```python
from build123d import *

# Parameters (mm, degrees)
F0_W      = 20
F0_H      = 5
F1_DEPTH  = 2
F2_R      = 2
F3_W      = 16
F3_H      = 2
F4_DEPTH  = 4
F5_R      = 2
F6_R      = 0.5
F7_DEPTH  = 2.001
F8_R      = 1.376408
F9_DEPTH  = 2.001
F11_W     = 1.233603
F11_H     = 9
F10_W     = 1.27
F10_H     = 9
F12_DEPTH = 0.635


with BuildPart() as f1:
    # F0 (on Top) → F1 (new body)
    with BuildSketch(Plane.XY):
        Rectangle(F0_W, F0_H)
    extrude(amount=F1_DEPTH)

    # F2
    f2_edges = [f1.edges().sort_by_distance(p)[0] for p in [
        (-10, -2.5, 1),
        (-10, 2.5, 1),
        (10, 2.5, 1),
        (10, -2.5, 1),
    ]]
    fillet(f2_edges, radius=F2_R)

    # F3 (on face) → F4 (join)
    with BuildSketch(Plane(origin=(0, 2.5, 0), x_dir=(-1, 0, 0), z_dir=(0, 1, 0))):
        with Locations((0, 1)):
            Rectangle(F3_W, F3_H)
    extrude(amount=F4_DEPTH)

    # F5
    f5_edges = [f1.edges().sort_by_distance(p)[0] for p in [
        (-8, 6.5, 1),
        (8, 6.5, 1),
    ]]
    fillet(f5_edges, radius=F5_R)

    # F6 (on face) → F7 (cut, through all)
    with BuildSketch(Plane.XY.offset(2)):
        Circle(F6_R)
        with Locations((-5, 0)):
            Circle(F6_R)
        with Locations((5, 0)):
            Circle(F6_R)
    extrude(amount=-F7_DEPTH, mode=Mode.SUBTRACT)

    # F8 (on face) → F9 (cut, through all)
    with BuildSketch(Plane.XY.offset(2)):
        with Locations((-7.627351, 0)):
            Circle(F8_R)
        with Locations((7.627366, 0)):
            Circle(F8_R)
        with Locations((-5, 3.96)):
            Circle(F8_R)
        with Locations((0, 3.96)):
            Circle(F8_R)
        with Locations((5, 3.96)):
            Circle(F8_R)
    extrude(amount=-F9_DEPTH, mode=Mode.SUBTRACT)

    # F11 (on face) + F10 (on face) → F12 (cut)
    with BuildSketch(Plane.XY.offset(2)):
        with Locations((-2.538401, 2)):
            Rectangle(F11_W, F11_H)
    with BuildSketch(Plane.XY.offset(2)):
        with Locations((2.54, 2)):
            Rectangle(F10_W, F10_H)
    extrude(amount=-F12_DEPTH, mode=Mode.SUBTRACT)


solid = f1.part
```
Geometry check sheet. Reference: the model listing, model coordinates, mm. A direction names the side the tool comes from. Give positions to 0.01 mm unless a question says otherwise; leave off trailing zeros. Loops run counter-clockwise (first coordinate to the right, second up) from the corner with the lowest first, then second, coordinate; pieces in that order, holes last. Notation, with made-up numbers: M -37,-4 L 14,-4 A31 cw 14,28 Z; hole C 25.25,74 d8. An arc over 180 degrees is marked long. Answer as CSV lines item,"result".
Item 1: Depth check by flat-ended pin: P1, Ø2, axis at x = 0, y = 3.96, coming from the -Z side; P2, Ø0.6, axis at y = 4, z = 1, coming from the +X side; P3, Ø1, axis at y = 4, z = 0.5, coming from the -X side. Enter the tip coordinate at first touch or a pass-through.
Values:
P1,"passes through"
P2,"stops at x = 8"
P3,"stops at x = -8"
Item 2: Access from +Z, -Z, +X, -X, +Y, -Y to the whole of each face (thin tool, end or side, straight path). Record for faces 1 (the cylindrical face through (8.899, -0.527, 1.014)), 2 (the flat face through (3, 2, 1.365)).
Values:
face 1,"+Z, -Z"
face 2,"+Z, +Y, -Y"
Item 3: Release check for a two-part mould opening along X. For faces 3 (the cylindrical face through (-0.298, 2.616, 1.014)), 4 (the cylindrical face through (-0.108, -0.488, 1.014)), 5 (the flat face through (-10, 0, 1)), 6 (the flat face through (0, -2.5, 1)) record: pulls with the +X half, pulls with the -X half, needs draft (parallel to the pull), parting line crosses it, or undercut.
Values:
face 3,"undercut"
face 4,"undercut"
face 5,"pulls with the -X half"
face 6,"needs draft"
Item 4: Cross-section at B-B on x = -5. Record the cut outline in (y, z).
Values:
outline,"M -2.5,0 L -0.5,0 L -0.5,2 L -2.5,2 Z; M 0.5,0 L 2.58,0 L 2.58,2 L 0.5,2 Z; M 5.34,0 L 6.5,0 L 6.5,2 L 5.34,2 Z"
Item 5: Cross-section at C-C on y = 0. Count the separate pieces of the cut face and the enclosed holes in it, and give its area (3 significant figures).
Values:
separate pieces,"6"
enclosed holes,"0"
area,"21.4 mm²"
Item 6: Material ranges on line 1 (Y direction, x = -5, z = 1.2); line 2 (Y direction, x = -5.25, z = 0.3); line 3 (X direction, y = 3.75, z = 0.45), recorded low to high.
Values:
line 1,"y = -2.5 to -0.5, 0.5 to 2.58, 5.34 to 6.5"
line 2,"y = -2.5 to -0.43, 0.43 to 2.61, 5.31 to 6.5"
line 3,"x = -8 to -6.36, -3.64 to -1.36, 1.36 to 3.64, 6.36 to 8"
Item 7: Cross-section at A-A on y = 3.96. Record the cut outline in (x, z) (3 decimals).
Values:
outline,"M -8,0 L -6.376,0 L -6.376,2 L -8,2 Z; M -3.624,0 L -1.376,0 L -1.376,2 L -1.922,2 L -1.922,1.365 L -3.155,1.365 L -3.155,2 L -3.624,2 Z; M 1.376,0 L 3.624,0 L 3.624,2 L 3.175,2 L 3.175,1.365 L 1.905,1.365 L 1.905,2 L 1.376,2 Z; M 6.376,0 L 8,0 L 8,2 L 6.376,2 Z"
